Input: part model. Units: mm. Frame: model coordinates. A direction names the side the tool comes from. Coordinates: 2 decimals unless noted, no trailing zeros. Order: outer loops, then holes, each group sorted by start corner. A loop starts at its lowest first (then second) coordinate and runs counter-clockwise, first axis right, second up. Notation, with made-up numbers: (19, 51.5) -> (37, 51.5) arc R24 cw to (37, 73.5) -> close; hole circle Ø1 at (44.5, -26). An arc over 180 degrees is marked (long way). One line per question, with ' | ' between items.
```python
from build123d import *

# Parameters (mm, degrees)
SKETCH1_R           = 1.5
BOSS_EXTRUDE1_DEPTH = 8.5
BOSS_EXTRUDE2_DEPTH = 8.5


with BuildPart() as part:
    # Sketch1 → Boss-Extrude1 (new body)
    with BuildSketch(Plane(origin=(0, 0, 0), x_dir=(0, 0, -1), z_dir=(1, 0, 0))):
        with BuildLine():
            Line((27, 10), (5, 10))
            ThreePointArc((5, 10), (0, 5), (5, 0))
            Line((5, 0), (27, 0))
            ThreePointArc((27, 0), (32, 5), (27, 10))
        make_face()
        with Locations((5, 5)):
            Circle(SKETCH1_R, mode=Mode.SUBTRACT)
        with Locations((27, 5)):
            Circle(SKETCH1_R, mode=Mode.SUBTRACT)
    extrude(amount=BOSS_EXTRUDE1_DEPTH)

    # Sketch2 → Boss-Extrude2 (add)
    with BuildSketch(Plane(origin=(8.5, 0, 0), x_dir=(0, 0, -1), z_dir=(1, 0, 0))):
        with BuildLine():
            ThreePointArc((27, 10), (29.863119288, 9.099091112), (31.69447473, 6.721019177))
            Line((31.69447473, 6.721019177), (31.867747629, 7.092604107))
            Line((31.867747629, 7.092604107), (45.02344432, 11.880886114))
            Line((45.02344432, 11.880886114), (51.43200814, 8.892523726))
            Line((51.43200814, 8.892523726), (60.828934348, 12.31272516))
            Line((60.828934348, 12.31272516), (57.408732915, 21.709651368))
            Line((57.408732915, 21.709651368), (25.236730193, 10))
            Line((25.236730193, 10), (27, 10))
        make_face()
        Polygon((60.828934348, 12.31272516), (51.43200814, 8.892523726), (51.774028284, 7.952831106), (61.170954492, 11.373032539), align=None)
    extrude(amount=-BOSS_EXTRUDE2_DEPTH)


solid = part.part
```
1. Cut plane B-B, the plane y = 5. Return loops of the section in (x, z), and give its area (3 significant figures).
Recorded:
outline: (0, -32) -> (8.5, -32) -> (8.5, -28.5) -> (0, -28.5) -> close; (0, -25.5) -> (8.5, -25.5) -> (8.5, -6.5) -> (0, -6.5) -> close; (0, -3.5) -> (8.5, -3.5) -> (8.5, 0) -> (0, 0) -> close | area: 221 mm^2
2. Cut plane C-C, the plane z = -48. Return loops of the section in (x, y).
Recorded:
outline: (0, 10.49) -> (8.5, 10.49) -> (8.5, 18.29) -> (0, 18.29) -> close
3. Cut plane A-A, the plane x = 7.5. Return loops of the section in (y, z), and give its area (3 significant figures).
Recorded:
outline: (0, -27) arc R5 ccw to (6.72, -31.69) -> (7.09, -31.87) -> (11.88, -45.02) -> (8.89, -51.43) -> (7.95, -51.77) -> (11.37, -61.17) -> (21.71, -57.41) -> (10, -25.24) -> (10, -5) arc R5 ccw to (0, -5) -> close; hole circle Ø3 at (5, -27); hole circle Ø3 at (5, -5) | area: 510 mm^2
4. Pin query (flat end, axial travel): pin 1 Ø1.5 at (x, z) = (3, -43.5) entering from +Y; pin 2 Ø4 at (x, z) = (5, -20) entering from +Y; pin 3 Ø5 at (x, y) = (5.5, 15) entering from -Z. Return the tip coordinate at first contact, or that it passes through.
Recorded:
pin 1: stops at y = 16.92 | pin 2: stops at y = 10 | pin 3: stops at z = -60.76
5. Access query for faces 1 (the face through (4, 2, -31)), 2 (the face through (4.3, 10.4, -48.2)). Directions: +Z, -Z, +X, -X, +Y, -Y. A direction counts if a zero-diameter tool reaches every point of the face in a straight line with its end or side. Return the directions, or none.
Recorded:
face 1: -Z, +X, -X | face 2: +X, -X, -Y
6. Ray query, line 1 (Y direction, x = 2.25, z = -5); line 2 (Y direction, x = 0.5, z = -15.5); line 3 (Y direction, x = 6.5, z = -27). Return the intervals inside material, ascending. Write a range as [from, to].
Recorded:
line 1: y = [0, 3.5], [6.5, 10] | line 2: y = [0, 10] | line 3: y = [0, 3.5], [6.5, 10.64]
7. Mould query, pull axis Z, two halves, no side actions, for faces 3 (the face through (4.19, 5.07, -25.5)), 4 (the face through (4, 10, -15)), 5 (the face through (4, 5, 0)). Classes: released by +Z, released by -Z, zero draft, split by the parting line, or undercut.
Recorded:
face 3: undercut | face 4: zero draft | face 5: released by +Z
8. Cut plane D-D, the plane y = 16.25. Return loops of the section in (x, z).
Recorded:
outline: (0, -59.4) -> (8.5, -59.4) -> (8.5, -42.41) -> (0, -42.41) -> close
